from build123d import *

# Parameters (mm, degrees)
SKETCH1_W           = 25.4
SKETCH1_H           = 1.5875
BOSS_EXTRUDE1_DEPTH = 5.588


with BuildPart() as part:
    # Sketch1 → Boss-Extrude1 (new body)
    # profile 1 of 3: a face of its own
    with BuildSketch(Plane(origin=(-94.488, 0, 0), x_dir=(0, -1, 0), z_dir=(-1, 0, 0))):
        Polygon((136.525, -196.85), (111.125, -196.85), (111.125, -203.2), (85.725, -203.2), (85.725, -196.85), (60.325, -196.85), (60.325, -682.625), (85.725, -682.625), (85.725, -679.45), (111.125, -679.45), (111.125, -682.625), (136.525, -682.625), align=None)
        with Locations((98.425, -456.40625)):
            Rectangle(SKETCH1_W, SKETCH1_H, mode=Mode.SUBTRACT)
    # profile 2 of 3: a face of its own
    with BuildSketch(Plane(origin=(-94.488, 0, 0), x_dir=(0, -1, 0), z_dir=(-1, 0, 0))):
        with BuildLine():
            Line((149.225, -203.2), (136.525, -203.2))
            Line((136.525, -203.2), (136.525, -290.406498707))
            ThreePointArc((136.525, -290.406498707), (137.30121982, -286.034603668), (139.534994681, -282.197126202))
            Line((139.534994681, -282.197126202), (184.118202659, -229.57294303))
            ThreePointArc((184.118202659, -229.57294303), (185.23509009, -227.654204297), (185.6232, -225.468256778))
            Line((185.6232, -225.468256778), (185.6232, -203.2))
            Line((185.6232, -203.2), (168.275, -203.2))
            Line((168.275, -203.2), (168.275, -196.85))
            Line((168.275, -196.85), (149.225, -196.85))
            Line((149.225, -196.85), (149.225, -203.2))
        make_face()
    # profile 3 of 3: a face of its own
    with BuildSketch(Plane(origin=(-94.488, 0, 0), x_dir=(0, -1, 0), z_dir=(-1, 0, 0))):
        with BuildLine():
            ThreePointArc((138.226477372, -606.197045256), (136.957742006, -603.134047129), (136.525, -599.847045256))
            Line((136.525, -599.847045256), (136.525, -679.45))
            Line((136.525, -679.45), (146.05, -679.45))
            Line((146.05, -679.45), (146.05, -684.2125))
            Line((146.05, -684.2125), (161.925, -684.2125))
            Line((161.925, -684.2125), (161.925, -679.45))
            Line((161.925, -679.45), (171.45, -679.45))
            Line((171.45, -679.45), (171.45, -665.443351826))
            ThreePointArc((171.45, -665.443351826), (171.233628997, -663.79985089), (170.599261314, -662.268351826))
            Line((170.599261314, -662.268351826), (138.226477372, -606.197045256))
        make_face()
    extrude(amount=-BOSS_EXTRUDE1_DEPTH)


solid = part.part
Read the model definition and answer for the solid it produces. Units are mm, in the model's axes. A direction names the side the tool comes from. Round coordinates to 2 decimals unless told otherwise and drop trailing zeros. Write each loop counter-clockwise with the first axis right and the second up, starting at its lowest first coordinate (ties: lowest second). Pieces come first, ordered by that corner, then holes. Notation, with made-up numbers: (57, 34) - (92, 34) arc R19 cw to (92, 57) - close; hole circle Ø11 at (58.5, -33.75). An arc over 180 degrees is marked (long way). One line per question, with ' | ' between items. Start each with the question number.
1. For a pull along Z with two mould halves and no side action, classify faces 3 (the face through (-94.488, -108, -437)), 4 (the face through (-91.73, -154.64, -634.63)) as +Z half, -Z half, draft (parallel to the pull), parting line (faces both ways), or undercut.
2. Find the intervals of material crossed by probe 1 along Z at (x, y) = (-93.95, -108); probe 2 along Z at (x, y) = (-92.9, -82) (3 decimals); probe 3 along Y at (x, z) = (-91.4, -452) (3 decimals), in increasing order. Write a range as [from, to].
3. Section C-C (y = -178) is taken. Determine the outline of the cut face in (x, z).
4. Section A-A (y = -103.5) is taken. Determine the outline of the cut face in (x, z), and give its area (3 significant figures).
5. Section B-B (z = -339.5) is taken. Determine the outline of the cut face in (x, y) (3 decimals), and give its area (3 significant figures).
6. For faces 1 (the face through (-91.733, -161.515, -256.253)), 2 (the face through (-88.9, -108, -437)), determine the directions among +Z, -Z, +X, -X, +Y, -Y from which every point of the face is accessible in a straight line to the end or side of a thin tool.
7. Each of these flat-tipped pins is pushed along its axis until it touches: pin 1 (1 mm diameter, centred on x = -91.5, y = -82, fed in from -Z) (3 decimals); pin 2 (1.7 mm diameter, centred on x = -92, z = -200, fed in from -Y) (3 decimals); pin 3 (0.8 mm diameter, centred on x = -90.5, z = -456.5, fed in from -Y) (3 decimals). Where does it stop, or does it pass through?
Filled in:
1) face 3: draft | face 4: undercut
2) probe 1: [-679.45, -457.2], [-455.61, -203.2] | probe 2: [-682.625, -196.85] | probe 3: [-136.525, -60.325]
3) outline: (-94.49, -236.79) - (-88.9, -236.79) - (-88.9, -203.2) - (-94.49, -203.2) - close
4) outline: (-94.49, -679.45) - (-88.9, -679.45) - (-88.9, -457.2) - (-94.49, -457.2) - close; (-94.49, -455.61) - (-88.9, -455.61) - (-88.9, -203.2) - (-94.49, -203.2) - close | area: 2,650 mm²
5) outline: (-94.488, -136.525) - (-88.9, -136.525) - (-88.9, -60.325) - (-94.488, -60.325) - close | area: 426 mm²
6) face 1: +X, -X, -Y | face 2: +Z, -Z, +X, +Y, -Y
7) pin 1: z = -682.625 | pin 2: y = -168.275 | pin 3: y = -136.525
